Here's how the part is built. I have some questions about the finished solid (model axes, mm). A direction names the side the tool comes from. Coordinates: 2 decimals unless noted, no trailing zeros. Order: outer loops, then holes, each group sorted by start corner. A loop starts at its lowest first (then second) coordinate and runs counter-clockwise, first axis right, second up.
```python
from build123d import *

# Parameters (mm, degrees)
SKETCH1_W           = 66
SKETCH1_H           = 5
BASE_FLANGE1_DEPTH  = 2
SKETCH2_R           = 2.5
BOSS_EXTRUDE1_DEPTH = 3
SKETCH3_W           = 2
SKETCH3_H           = 5
BOSS_EXTRUDE2_DEPTH = 11
SKETCH4_W           = 6
SKETCH4_H           = 5
BOSS_EXTRUDE3_DEPTH = 2
SKETCH5_R           = 1.5
CUT_EXTRUDE1_DEPTH  = 40.537956447
SKETCH6_R           = 1.25
CUT_EXTRUDE2_DEPTH  = 41.598645298
SKETCH7_W           = 2
SKETCH7_H           = 5
BOSS_EXTRUDE4_DEPTH = 25
BOSS_EXTRUDE5_DEPTH = 5


# Sheet-metal steps are written as plain solids
with BuildPart() as part:
    # Sketch1 → Base-Flange1 (new body)
    with BuildSketch(Plane(origin=(0, 0, 0), x_dir=(1, 0, 0), z_dir=(0, 1, 0))):
        Rectangle(SKETCH1_W, SKETCH1_H)
    extrude(amount=-BASE_FLANGE1_DEPTH)

    # Sketch2 → Boss-Extrude1 (add)
    with BuildSketch(Plane(origin=(0, 0, 0), x_dir=(-1, 0, 0), z_dir=(0, -1, 0))):
        with Locations(Location((19.7, 0, 0), (0, 0, 90))):
            Circle(SKETCH2_R)
        with Locations(Location((-29.3, 0, 0), (0, 0, 90))):
            Circle(SKETCH2_R)
    extrude(amount=-BOSS_EXTRUDE1_DEPTH)

    # Sketch3 → Boss-Extrude2 (add)
    with BuildSketch(Plane(origin=(0, -2, 0), x_dir=(-1, 0, 0), z_dir=(0, -1, 0))):
        with Locations((-34, 0)):
            Rectangle(SKETCH3_W, SKETCH3_H)
    boss_extrude2 = extrude(amount=-BOSS_EXTRUDE2_DEPTH)

    # Sketch4 → Boss-Extrude3 (add)
    with BuildSketch(Plane(origin=(0, 9, 0), x_dir=(1, 0, 0), z_dir=(0, 1, 0))):
        with Locations((36, 0)):
            Rectangle(SKETCH4_W, SKETCH4_H)
    boss_extrude3 = extrude(amount=-BOSS_EXTRUDE3_DEPTH)

    # Mirror1: Boss-Extrude2, Boss-Extrude3 across plane
    add(boss_extrude2.mirror(Plane(origin=(0, 0, 0), x_dir=(0, 0, 1), z_dir=(1, 0, 0))))
    add(boss_extrude3.mirror(Plane(origin=(0, 0, 0), x_dir=(0, 0, 1), z_dir=(1, 0, 0))))

    # Sketch5 → Cut-Extrude1 (cut, through all)
    with BuildSketch(Plane(origin=(0, 3, 0), x_dir=(1, 0, 0), z_dir=(0, 1, 0))):
        with Locations(Location((-19.7, 0, 0), (0, 0, 270))):
            Circle(SKETCH5_R)
        with Locations(Location((29.3, 0, 0), (0, 0, 270))):
            Circle(SKETCH5_R)
    extrude(amount=-CUT_EXTRUDE1_DEPTH, mode=Mode.SUBTRACT)

    # Sketch6 → Cut-Extrude2 (cut, through all)
    with BuildSketch(Plane(origin=(0, 9, 0), x_dir=(1, 0, 0), z_dir=(0, 1, 0))):
        with Locations(Location((-37, 0, 0), (0, 0, 270))):
            Circle(SKETCH6_R)
        with Locations(Location((37, 0, 0), (0, 0, 270))):
            Circle(SKETCH6_R)
    extrude(amount=-CUT_EXTRUDE2_DEPTH, mode=Mode.SUBTRACT)

    # Sketch7 → Boss-Extrude4 (add)
    with BuildSketch(Plane(origin=(0, -2, 0), x_dir=(-1, 0, 0), z_dir=(0, -1, 0))):
        with Locations((29, 0)):
            Rectangle(SKETCH7_W, SKETCH7_H)
    boss_extrude4 = extrude(amount=BOSS_EXTRUDE4_DEPTH)

    # Sketch8 → Boss-Extrude5 (add)
    with BuildSketch(Plane.XY.offset(2.5)):
        Polygon((-28, -3), (-26, -5), (-28, -5), align=None)
        Polygon((-28, -7), (-26, -7), (-28, -9), align=None)
        Polygon((-28, -21), (-28, -23), (-26, -23), align=None)
        Polygon((-28, -25), (-28, -27), (-26, -25), align=None)
    boss_extrude5 = extrude(amount=-BOSS_EXTRUDE5_DEPTH)

    # Mirror2: Boss-Extrude4, Boss-Extrude5 across plane
    add(boss_extrude4.mirror(Plane(origin=(2.5, 0, 0), x_dir=(0, 0, 1), z_dir=(1, 0, 0))))
    add(boss_extrude5.mirror(Plane(origin=(2.5, 0, 0), x_dir=(0, 0, 1), z_dir=(1, 0, 0))))


solid = part.part
```
Q1. If we section it at A-A on x = 37: Write out the boundary of the cut face in (y, z), then the cut area to 3 significant figures.
Q2. If we section it at D-D on z = 0.05: Give the number of separate pieces and of enclosed holes in the cut face, then the cut area to 3 significant figures.
Q3. If we section it at B-B on y = -14.5: Write out the boundary of the cut face in (x, z), then the cut area to 3 significant figures.
Q4. I need wall thicknesses on L1, parallel to X at y = 7.9, z = 0; L2, parallel to X at y = 0.6, z = 0; L3, parallel to X at y = -0.15, z = 0. Which ranges of each line are inside material? Lowest first, please.
Q5. We'd pull the mould along X, two halves only. Please class faces 1 (the flat face through (-28, -15, 0)), 2 (the flat face through (-39, 8, 0)), 3 (the flat face through (-36, 7, -1)): pulls with the +X half, pulls with the -X half, needs draft (parallel to the pull), parting line crosses it, or undercut.
Q6. For faces 4 (the flat face through (-30, -14, 0)), 5 (the flat face through (-28, -24, 0)), 6 (the flat face through (36, 7, -1)), 7 (the flat face through (33, 4, 0)), which set-ups out of +Z, -Z, +X, -X, +Y, -Y let a thin tool reach every point of the face, with its end or its side?
Q7. Will these pins go through, and if not, where does the flat tip stop? pin 1 (12 mm diameter, centred on x = -16.5, y = -7.5, fed in from +Z); pin 2 (1 mm diameter, centred on y = -6, z = 0.5, fed in from +X); pin 3 (3 mm diameter, centred on x = -37, z = -1, fed in from -Y); pin 4 (1.6 mm diameter, centred on x = 31.5, z = 0, fed in from -Y).
Q8. If we section it at C-C on x = 28.5: Write out the boundary of the cut face in (y, z), then the cut area to 3 significant figures.
Reply:
1. outline: (7, -2.5) - (9, -2.5) - (9, -1.25) - (7, -1.25) - close; (7, 1.25) - (9, 1.25) - (9, 2.5) - (7, 2.5) - close
1. area: 5.00 mm2
2. separate pieces: 5
2. enclosed holes: 0
2. area: 298 mm2
3. outline: (-30, -2.5) - (-28, -2.5) - (-28, 2.5) - (-30, 2.5) - close; (33, -2.5) - (35, -2.5) - (35, 2.5) - (33, 2.5) - close
3. area: 20.0 mm2
4. L1: x = -39 to -38.25, -35.75 to -33, 33 to 35.75, 38.25 to 39
4. L2: x = -35 to -33, -22.2 to -21.2, -18.2 to -17.2, 26.8 to 27.8, 30.8 to 31.8, 33 to 35
4. L3: x = -35 to -21.2, -18.2 to 27.8, 30.8 to 35
5. face 1: undercut
5. face 2: pulls with the -X half
5. face 3: needs draft
6. face 4: +Z, -Z, -X, -Y
6. face 5: +Z, -Z
6. face 6: +Z, -Z, +X, -Y
6. face 7: +Z, -Z, +Y
7. pin 1: stops at z = 2.5
7. pin 2: stops at x = 35
7. pin 3: stops at y = 7
7. pin 4: stops at y = -26.3
8. outline: (-2, -2.5) - (0, -2.5) - (0, -2.37) - (3, -2.37) - (3, -1.27) - (-2, -1.27) - close; (-2, 1.27) - (3, 1.27) - (3, 2.37) - (0, 2.37) - (0, 2.5) - (-2, 2.5) - close
8. area: 11.5 mm2
